```python
from build123d import *

# Parameters (mm, degrees)
SKETCH001_R       = 0.95
PAD001_DEPTH      = 18.415
PAD001_DEPTH_BACK = 3.5
SKETCH_R          = 20.32
SKETCH_R_2        = 2.225
PAD_DEPTH         = 36.83
FILLET_R          = 0.5


with BuildPart() as pad001:
    # Sketch001 → Pad001 (new body, two sides)
    with BuildSketch(Plane.XY.offset(0.5)) as pad001_sk:
        Circle(SKETCH001_R)
        with Locations((27.94, 0)):
            Circle(SKETCH001_R)
    extrude(amount=PAD001_DEPTH)
    extrude(pad001_sk.sketch, amount=-PAD001_DEPTH_BACK)


with BuildPart() as obj1:
    # Sketch → Pad (new body)
    with BuildSketch(Plane.XY.offset(0.1)):
        with Locations((13.97, 0)):
            Circle(SKETCH_R)
        with Locations((13.97, 0)):
            Circle(SKETCH_R_2, mode=Mode.SUBTRACT)
    extrude(amount=PAD_DEPTH)

    # Fillet
    fillet_edges = [obj1.edges().sort_by_distance(p)[0] for p in [
        (11.745, 0, 36.93),
        (-6.35, 0, 36.93),
        (-6.35, 0, 0.1),
    ]]
    fillet(fillet_edges, radius=FILLET_R)

    # obj1: union Pad001
    add(pad001.part)


solid = obj1.part
```
Read the model definition and answer for the solid it produces. Units are mm, in the model's axes. A direction names the side the tool comes from. Give positions to 0.01 mm unless a question says otherwise; leave off trailing zeros. Write each loop counter-clockwise with the first axis right and the second up, starting at its lowest first coordinate (ties: lowest second). Pieces come first, ordered by that corner, then holes. Notation, with made-up numbers: (-0.5, -6.5) -> (40.5, -6.5) arc R25 ccw to (40.5, 25.5) -> close; hole circle Ø6 at (-17, 44.5). An arc over 180 degrees is marked (long way). Answer in a Markdown table with one row per item.
1) Straight lines are drawn through the part: line 1 (Y direction, x = 13.97, z = 15) (3 decimals); line 2 (Z direction, x = 25, y = 16); line 3 (Y direction, x = 13, z = 21.5). For each, find the intervals that lie inside material, in ascending order. Write a range as [from, to].
Results list:
| item | result |
|---|---|
| line 1 | [-20.32, -2.225], [2.225, 20.32] |
| line 2 | [0.1, 36.93] |
| line 3 | [-20.3, -2], [2, 20.3] |
2) Each of these flat-tipped pins is pushed along its axis until it touches: pin 1 Ø6 at (x, z) = (-2, 15) entering from +Y; pin 2 Ø12 at (x, y) = (19, -8.5) entering from -Z; pin 3 Ø8 at (x, z) = (7.5, 17) entering from -Y. Where does it stop, or does it pass through?
Results list:
| item | result |
|---|---|
| pin 1 | y = 15.64 |
| pin 2 | z = 0.1 |
| pin 3 | y = -20.17 |
3) Determine the mould class of faces 3 (the cylindrical face through (12.2, -1.35, 18.01)), 4 (the cylindrical face through (-0.95, 0.04, -1.43)), 5 (the flat face through (14, -4, 36.93)) for opening direction Y: released by +Y, released by -Y, zero draft, split by the parting line, or undercut.
Results list:
| item | result |
|---|---|
| face 3 | undercut |
| face 4 | split by the parting line |
| face 5 | zero draft |
4) Section B-B on y = 0 is taken. Give the vertices of the cut face in (x, z) (3 decimals), plus the area to 3 significant figures.
Results list:
| item | result |
|---|---|
| outline | (-6.35, 0.6) arc R0.5 ccw to (-5.85, 0.1) -> (-0.95, 0.1) -> (-0.95, -3) -> (0.95, -3) -> (0.95, 0.1) -> (11.745, 0.1) -> (11.745, 36.43) arc R0.5 ccw to (11.245, 36.93) -> (-5.85, 36.93) arc R0.5 ccw to (-6.35, 36.43) -> close; (16.195, 0.1) -> (26.99, 0.1) -> (26.99, -3) -> (28.89, -3) -> (28.89, 0.1) -> (33.79, 0.1) arc R0.5 ccw to (34.29, 0.6) -> (34.29, 36.43) arc R0.5 ccw to (33.79, 36.93) -> (16.695, 36.93) arc R0.5 ccw to (16.195, 36.43) -> close |
| area | 1,340 mm^2 |
5) A tool of negligible diameter and unlimited length cuts with its end or side. For faces 1 (the cylindrical face through (28.846, 0.285, -1.428)), 2 (the flat face through (0, 0, -3)), from which of +Z, -Z, +X, -X, +Y, -Y can it reach the whole face along a straight path? Write none if from no direction.
Results list:
| item | result |
|---|---|
| face 1 | -Z |
| face 2 | -Z, +X, -X, +Y, -Y |
6) Section A-A on x = 13.97 is taken. Give the vertices of the cut face in (y, z) (3 decimals), plus the area to 3 significant figures.
Results list:
| item | result |
|---|---|
| outline | (-20.32, 0.6) arc R0.5 ccw to (-19.82, 0.1) -> (-2.225, 0.1) -> (-2.225, 36.43) arc R0.5 ccw to (-2.725, 36.93) -> (-19.82, 36.93) arc R0.5 ccw to (-20.32, 36.43) -> close; (2.225, 0.1) -> (19.82, 0.1) arc R0.5 ccw to (20.32, 0.6) -> (20.32, 36.43) arc R0.5 ccw to (19.82, 36.93) -> (2.725, 36.93) arc R0.5 ccw to (2.225, 36.43) -> close |
| area | 1,330 mm^2 |
7) Section C-C on z = 3.5 is taken. Give the vertices of the cut face in (x, y) (3 decimals).
Results list:
| item | result |
|---|---|
| outline | circle Ø40.64 at (13.97, 0); hole circle Ø4.45 at (13.97, 0) |
